Source: CAD feature listing. Evaluate the final solid. Frame: model axes, mm. A direction names the side the tool comes from. Coordinates: 2 decimals unless noted, no trailing zeros. Order: outer loops, then holes, each group sorted by start corner. A loop starts at its lowest first (then second) coordinate and runs counter-clockwise, first axis right, second up. Notation, with made-up numbers: (-4, 26) - (5, 26) arc R12 ccw to (5, 37) - close; hole circle Ø1 at (27, 9.5). An arc over 180 degrees is marked (long way). One line per question, with ' | ' between items. Start each with the question number.
(1) Section C-C (y = -31). Return the cut outline in (x, z), then the cut area to 3 significant figures.
(2) Access query for faces 1 (the flat face through (-24.452, -21, 7)), 2 (the flat face through (-16, -1, 0)). Directions: +Z, -Z, +X, -X, +Y, -Y. A direction counts if a zero-diameter tool reaches every point of the face in a straight line with its end or side. Return the directions, or none.
(3) Line query: line 1 along X through (y, z) = (7, 8); line 2 along Y through (x, z) = (-13, 8.75); line 3 along X through (y, z) = (-21, 13.25). Output: solid intervals per line, ascending.
(4) Draft query along Y for faces 3 (the flat face through (45.548, 7, 7)), 4 (the cylindrical face through (34.264, 8.273, 6.059)), 5 (the flat face through (-4, 19.658, 7)), 6 (the cylindrical face through (-40.34, 8.55, 6.06)). Return one class per face: +Y half, -Y half, draft (parallel to the pull), parting line (faces both ways), or undercut.
(5) Section A-A (z = 6.25). Return the cut outline in (x, y).
(6) Contact query for flat-ended pins moving along their axis: P1, Ø1, axis at x = -8, z = 11, coming from the -Y side; P2, Ø7, axis at y = -27, z = 6, coming from the +X side. Output: stop coordinate, or through.
(7) Section B-B (x = 40.5). Return the cut outline in (y, z), then the cut area to 3 significant figures.
from build123d import *

# Parameters (mm, degrees)
F1_DEPTH       = 14
F3_D           = 3.3
F3_CSINK_D     = 6.72
F3_CSINK_ANGLE = 90


with BuildPart() as f1:
    # F0 (on Top) → F1 (new body)
    with BuildSketch(Plane.XY):
        Polygon((45.5477632582, 19.6576939523), (-54.4522367418, 19.6576939523), (-54.4522367418, -35.3423060477), (-24.4522367418, -35.3423060477), (-24.4522367418, -5.3423060477), (45.5477632582, -5.3423060477), align=None)
    extrude(amount=F1_DEPTH)

    # F3 (through all)
    with Locations(Plane.XY.offset(14)):
        with Locations((-39.4522367418, 7.1576939523), (33.0477632582, 7.1576939523)):
            CounterSinkHole(F3_D / 2, F3_CSINK_D / 2, counter_sink_angle=F3_CSINK_ANGLE)


solid = f1.part
Response values:
1) outline: (-54.45, 0) - (-24.45, 0) - (-24.45, 14) - (-54.45, 14) - close | area: 420 mm²
2) face 1: +Z, -Z, +X, -Y | face 2: -Z, +X, -X, +Y, -Y
3) line 1: x = -54.45 to -41.09, -37.81 to 31.41, 34.69 to 45.55 | line 2: y = -5.34 to 19.66 | line 3: x = -54.45 to -24.45
4) face 3: draft | face 4: undercut | face 5: +Y half | face 6: undercut
5) outline: (-54.45, -35.34) - (-24.45, -35.34) - (-24.45, -5.34) - (45.55, -5.34) - (45.55, 19.66) - (-54.45, 19.66) - close; hole circle Ø3.3 at (-39.45, 7.16); hole circle Ø3.3 at (33.05, 7.16)
6) P1: stops at y = -5.34 | P2: stops at x = -24.45
7) outline: (-5.34, 0) - (19.66, 0) - (19.66, 14) - (-5.34, 14) - close | area: 350 mm²
